```python
from build123d import *

# Parameters (mm, degrees)
BOSS_EXTRUDE1_DEPTH       = 6
CUT_EXTRUDE1_DEPTH        = 102.003801713
CUT_EXTRUDE2_DEPTH        = 3
F_2_CLEARANCE_HOLE1_D     = 2.5
F_1_1_8_CLEARANCE_HOLE1_D = 29
F_3_CLEARANCE_HOLE1_D     = 3
FILLET1_R                 = 2
FILLET2_R                 = 3
FILLET3_R                 = 10
SKETCH10_R                = 27.5
CUT_EXTRUDE3_DEPTH        = 2.5
FILLET4_R                 = 1


with BuildPart() as part:
    # Sketch1 → Boss-Extrude1 (new body)
    with BuildSketch(Plane.XY.offset(6)):
        with BuildLine():
            Line((74.569864729, 20.944878138), (8.930118766, 20.944878138))
            ThreePointArc((8.930118766, 20.944878138), (5.269864729, 24.605132176), (0.269864729, 25.944878138))
            Line((0.269864729, 25.944878138), (-97.430135271, 25.944878138))
            Line((-97.430135271, 25.944878138), (-97.430135271, -24.055121862))
            Line((-97.430135271, -24.055121862), (0.269864729, -24.055121862))
            ThreePointArc((0.269864729, -24.055121862), (5.269864729, -22.7153759), (8.930118767, -19.055121862))
            Line((8.930118767, -19.055121862), (74.569864729, -19.055121862))
            ThreePointArc((74.569864729, -19.055121862), (94.569864729, 0.944878138), (74.569864729, 20.944878138))
        make_face()
    extrude(amount=-BOSS_EXTRUDE1_DEPTH)

    # Sketch2 → Cut-Extrude1 (cut, through all)
    with BuildSketch(Plane(origin=(0, 0, 0), x_dir=(-1, 0, 0), z_dir=(0, 0, -1))):
        with BuildLine():
            Line((92.030135271, 20.944878138), (-3.269864729, 20.944878138))
            Line((-3.269864729, 20.944878138), (-3.269864729, -19.055121862))
            Line((-3.269864729, -19.055121862), (92.030135271, -19.055121862))
            Line((92.030135271, -19.055121862), (92.030135271, -6.985443419))
            ThreePointArc((92.030135271, -6.985443419), (93.930135271, 0.944878138), (92.030135271, 8.875199695))
            Line((92.030135271, 8.875199695), (92.030135271, 20.944878138))
        make_face()
    extrude(amount=-CUT_EXTRUDE1_DEPTH, mode=Mode.SUBTRACT)

    # Sketch3 → Cut-Extrude2 (cut)
    with BuildSketch(Plane.XY.offset(6)):
        with BuildLine():
            Line((74.569864729, 16.194878138), (3.269864729, 16.194878138))
            Line((3.269864729, 16.194878138), (3.269864729, -14.305121862))
            Line((3.269864729, -14.305121862), (74.569864729, -14.305121862))
            ThreePointArc((74.569864729, -14.305121862), (89.819864729, 0.944878138), (74.569864729, 16.194878138))
        make_face()
    extrude(amount=-CUT_EXTRUDE2_DEPTH, mode=Mode.SUBTRACT)

    # #2 Clearance Hole1 (through all)
    with Locations(Plane.XY.offset(6)):
        with Locations((49.569864729, 18.194878138), (19.569864729, -16.305121862), (19.569864729, 18.194878138), (49.569864729, -16.305121862)):
            Hole(F_2_CLEARANCE_HOLE1_D / 2)

    # 1-1/8 Clearance Hole1 (through all)
    with Locations(Plane.XY.offset(3)):
        with Locations((74.569864729, 0.944878138)):
            Hole(F_1_1_8_CLEARANCE_HOLE1_D / 2)

    # #3 Clearance Hole1 (through all)
    with Locations(Plane.XY.offset(6)):
        with Locations((-3.580135271, 23.444878138), (-43.580135271, 23.444878138), (-83.580135271, 23.444878138), (-94.530135271, 12.944878138), (-94.530135271, -11.055121862), (-43.580135271, -21.555121862), (-3.580135271, -21.555121862), (-83.580135271, -21.555121862)):
            Hole(F_3_CLEARANCE_HOLE1_D / 2)

    # Fillet1
    fillet1_edges = [part.edges().sort_by_distance(p)[0] for p in [
        (3.269864729, -19.055121862, 3),
        (3.269864729, 20.944878138, 3),
    ]]
    fillet(fillet1_edges, radius=FILLET1_R)

    # Fillet2
    fillet2_edges = [part.edges().sort_by_distance(p)[0] for p in [
        (-92.030135271, 20.944878138, 3),
        (-92.030135271, -19.055121862, 3),
    ]]
    fillet(fillet2_edges, radius=FILLET2_R)

    # Fillet3
    fillet3_edges = [part.edges().sort_by_distance(p)[0] for p in [
        (-97.430135271, -24.055121862, 3),
        (-97.430135271, 25.944878138, 3),
    ]]
    fillet(fillet3_edges, radius=FILLET3_R)

    # Sketch10 → Cut-Extrude3 (cut)
    with BuildSketch(Plane(origin=(0, 0, 0), x_dir=(-1, 0, 0), z_dir=(0, 0, -1))):
        with Locations((-74.569864729, 0.944878138)):
            Circle(SKETCH10_R)
    extrude(amount=-CUT_EXTRUDE3_DEPTH, mode=Mode.SUBTRACT)

    # Fillet4
    fillet4_edges = [part.edges().sort_by_distance(p)[0] for p in [
        (55.695278641, -19.055121862, 1.25),
        (55.695278641, 20.944878138, 1.25),
    ]]
    fillet(fillet4_edges, radius=FILLET4_R)


solid = part.part
```
Check sheet for the modelled part. Datum: model origin and axes. Units: mm. A direction names the side the tool comes from. Give positions to 0.01 mm unless a question says otherwise; leave off trailing zeros. Order: outer loops, then holes, each group sorted by start corner. A loop starts at its lowest first (then second) coordinate and runs counter-clockwise, first axis right, second up. Notation, with made-up numbers: M 64.5,82.25 L 74.5,82.25 A33 cw 74.5,111.25 Z; hole C 27,38.5 d2. An arc over 180 degrees is marked long. Answer in a Markdown table with one row per item.
1) Cross-section at B-B, the plane y = 5. Enter the section's corners in (x, z), plus the area to 3 significant figures.
Filled sheet:
| item | result |
|---|---|
| outline | M -97.43,0 L -93.45,0 L -93.45,6 L -97.43,6 Z; M 3.27,0 L 47.37,0 L 47.37,2.5 L 60.65,2.5 L 60.65,3 L 3.27,3 Z; M 88.49,2.5 L 94.15,2.5 L 94.15,6 L 89.27,6 L 89.27,3 L 88.49,3 Z |
| area | 180 mm2 |
2) Cross-section at C-C, the plane x = 37. Enter the section's corners in (y, z).
Filled sheet:
| item | result |
|---|---|
| outline | M -19.06,0 L 20.94,0 L 20.94,6 L 16.19,6 L 16.19,3 L -14.31,3 L -14.31,6 L -19.06,6 Z |
3) Release check for a two-part mould opening along Y. For faces 1 (the flat face through (-44, -24.055, 3)), 2 (the flat face through (35, 20.945, 3)), 3 (the flat face through (36, 1, 3)) record: +Y half, -Y half, draft (parallel to the pull), parting line (faces both ways), or undercut.
Filled sheet:
| item | result |
|---|---|
| face 1 | -Y half |
| face 2 | +Y half |
| face 3 | undercut |
4) Thickness scan on L1, parallel to Y at x = -86, z = 0.45; L2, parallel to Y at x = 74, z = 4.7; L3, parallel to X at y = 22.5, z = 0.35. Record the ranges inside material, lowest first. Write a range as [from, to].
Filled sheet:
| item | result |
|---|---|
| L1 | y = [-24.06, -19.06], [20.94, 25.94] |
| L2 | y = [-19.06, -14.31], [16.19, 20.94] |
| L3 | x = [-94.98, -84.75], [-82.42, -44.75], [-42.42, -4.75], [-2.42, 7.82] |
5) Cross-section at D-D, the plane z = 0.9. Count the separate pieces of the cut face and the enclosed holes in it, plus the area to 3 significant figures.
Filled sheet:
| item | result |
|---|---|
| separate pieces | 1 |
| enclosed holes | 13 |
| area | 2,980 mm2 |
6) Cross-section at A-A, the plane x = -78. Enter the section's corners in (y, z).
Filled sheet:
| item | result |
|---|---|
| outline | M -24.06,0 L -19.06,0 L -19.06,6 L -24.06,6 Z; M 20.94,0 L 25.94,0 L 25.94,6 L 20.94,6 Z |
7) Access from +Z, -Z, +X, -X, +Y, -Y to the whole of each face (thin tool, end or side, straight path). Record for faces 4 (the cylindrical face through (47.07, 0.66, 1.23)), 5 (the cylindrical face through (-93.93, 0.83, 2.96)), 6 (the cylindrical face through (5.21, -22.75, 3.04)), 7 (the cylindrical face through (89.816, 0.61, 4.521)), 8 (the cylindrical face through (5.33, 24.57, 3.04)).
Filled sheet:
| item | result |
|---|---|
| face 4 | -Z, +X |
| face 5 | +Z, -Z |
| face 6 | +Z, -Z, +X, -Y |
| face 7 | +Z |
| face 8 | +Z, -Z, +X, +Y |
8) Gauge pin test, flat ends, axial feed: P1, Ø3, axis at x = 34, z = 2, coming from the -Y side; P2, Ø3.5, axis at x = -83.58, y = -21.56, coming from the +Z side; P3, Ø2.5, axis at x = -94.53, y = 12.94, coming from the -Z side; P4, Ø1.8, axis at y = -13, z = 3.5, coming from the +X side. Record the tip position at first contact, or that the pin passes through.
Filled sheet:
| item | result |
|---|---|
| P1 | stops at y = -19.06 |
| P2 | stops at z = 6 |
| P3 | passes through |
| P4 | stops at x = 89.73 |
